Input: dimensioned drawing with shaded views. Units: mm. Origin: part minimum x, y, z. A direction names the side the tool comes from. Give positions to 0.01 mm unless a question says otherwise; leave off trailing zeros. Write each loop counter-clockwise with the first axis right and the second up, starting at its lowest first coordinate (ties: lowest second). Pieces come first, ordered by that corner, then holes.
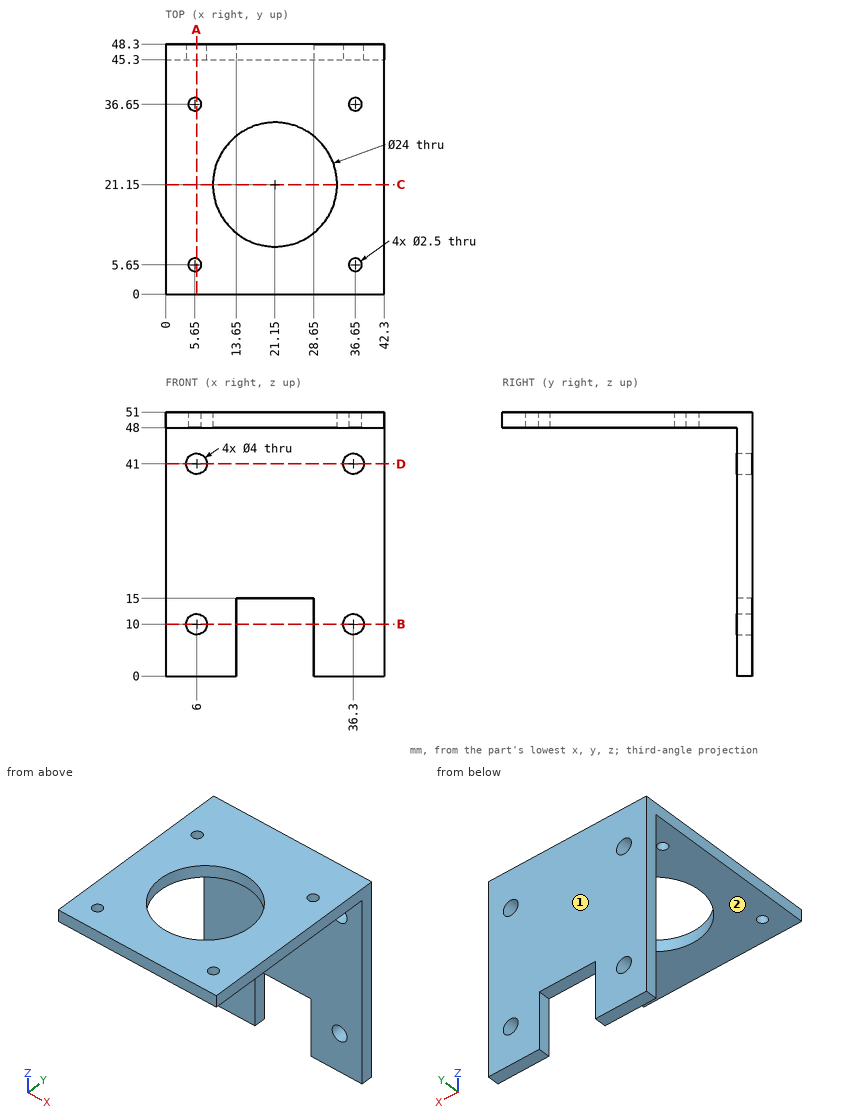
Item 1: Section A-A, the plane x = 6. Return the cut outline in (y, z).
Found:
outline: (0, 48) - (4.45, 48) - (4.45, 51) - (0, 51) - close; (6.85, 48) - (35.45, 48) - (35.45, 51) - (6.85, 51) - close; (37.85, 48) - (45.3, 48) - (45.3, 43) - (48.3, 43) - (48.3, 51) - (37.85, 51) - close; (45.3, 0) - (48.3, 0) - (48.3, 8) - (45.3, 8) - close; (45.3, 12) - (48.3, 12) - (48.3, 39) - (45.3, 39) - close
Item 2: Section D-D, the plane z = 41. Return the cut outline in (x, y), plus the area to 3 significant figures.
Found:
outline: (0, 45.3) - (4, 45.3) - (4, 48.3) - (0, 48.3) - close; (8, 45.3) - (34.3, 45.3) - (34.3, 48.3) - (8, 48.3) - close; (38.3, 45.3) - (42.3, 45.3) - (42.3, 48.3) - (38.3, 48.3) - close
area: 103 mm2
Item 3: Reachability of the marked faces 1 and 2 from +Z, -Z, +X, -X, +Y, -Y: full face, straight path, thin tool, end or side. Return the list, or none.
Found:
face 1: +Z, -Z, +X, -X, +Y
face 2: -Z, +X, -X, -Y
Item 4: Section C-C, the plane y = 21.15. Return the cut outline in (x, z).
Found:
outline: (0, 48) - (9.15, 48) - (9.15, 51) - (0, 51) - close; (33.15, 48) - (42.3, 48) - (42.3, 51) - (33.15, 51) - close
Item 5: Line query: L1, parallel to Z at x = 6, y = 46; L2, parallel to X at y = 21, z = 49; L3, parallel to Z at x = 34, y = 21.5. Output: solid intervals per line, ascending.
Found:
L1: z = 0 to 8, 12 to 39, 43 to 51
L2: x = 0 to 9.15, 33.15 to 42.3
L3: z = 48 to 51
Item 6: Pin query (flat end, axial travel): pin 1 Ø8 at (x, z) = (14, 15.5) entering from -Y; pin 2 Ø2 at (x, y) = (5.65, 36.65) entering from +Z; pin 3 Ø3 at (x, y) = (5.65, 5.65) entering from -Z; pin 4 Ø1.5 at (x, y) = (18, 46.5) entering from -Z. Return the tip coordinate at first contact, or that it passes through.
Found:
pin 1: stops at y = 45.3
pin 2: passes through
pin 3: stops at z = 48
pin 4: stops at z = 15
Item 7: Section B-B, the plane z = 10. Return the cut outline in (x, y), plus the area to 3 significant figures.
Found:
outline: (0, 45.3) - (4, 45.3) - (4, 48.3) - (0, 48.3) - close; (8, 45.3) - (13.65, 45.3) - (13.65, 48.3) - (8, 48.3) - close; (28.65, 45.3) - (34.3, 45.3) - (34.3, 48.3) - (28.65, 48.3) - close; (38.3, 45.3) - (42.3, 45.3) - (42.3, 48.3) - (38.3, 48.3) - close
area: 57.9 mm2
